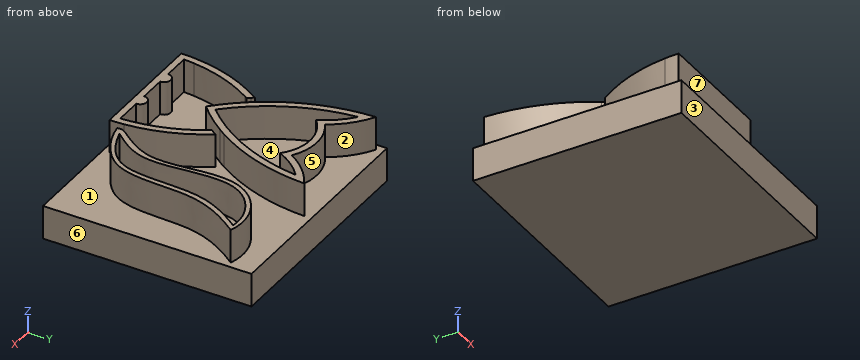
from build123d import *

# Parameters (mm, degrees)
F0_W     = 40
F0_H     = 40
F1_DEPTH = 5
F3_DEPTH = 5
F5_DEPTH = 5
F7_DEPTH = 5


with BuildPart() as f1:
    # F0 (on Top) → F1 (new body)
    with BuildSketch(Plane.XY):
        with Locations((0, -1.4423078379)):
            Rectangle(F0_W, F0_H)
    extrude(amount=F1_DEPTH)

    # F2 (on face) → F3 (join)
    with BuildSketch(Plane.XY.offset(5)):
        with BuildLine():
            ThreePointArc((-14.1666666667, 12.7937878067), (-16.2497421132, 15.4842249108), (-18.9811853554, 17.5132327819))
            ThreePointArc((-18.9811853554, 17.5132327819), (-17.6558893012, 9.8311930383), (-14.3321956463, 2.7797247698))
            ThreePointArc((-14.3321956463, 2.7797247698), (-14.0384410091, 2.335690009), (-13.7365842266, 1.8971228665))
            ThreePointArc((-13.7365842266, 1.8971228665), (-11.9756652837, -0.3650490595), (-10, -2.4423078379))
            ThreePointArc((-10, -2.4423078379), (-8.0243347163, -0.3650490595), (-6.2634157734, 1.8971228665))
            ThreePointArc((-6.2634157734, 1.8971228665), (-5.9615589909, 2.335690009), (-5.6678043537, 2.7797247698))
            ThreePointArc((-5.6678043537, 2.7797247698), (-2.3441106988, 9.8311930383), (-1.0188146446, 17.5132327819))
            ThreePointArc((-1.0188146446, 17.5132327819), (-3.7502578868, 15.4842249108), (-5.8333333333, 12.7937878067))
            ThreePointArc((-5.8333333333, 12.7937878067), (-10, 14.0576921621), (-14.1666666667, 12.7937878067))
        make_face()
        with BuildLine():
            ThreePointArc((-17.8386090668, 15.5557186069), (-15.9104422617, 13.6025441919), (-14.5, 11.2481079219))
            ThreePointArc((-14.5, 11.2481079219), (-10, 13.0576921621), (-5.5, 11.2481079219))
            ThreePointArc((-5.5, 11.2481079219), (-4.0895577383, 13.6025441919), (-2.1613909332, 15.5557186069))
            ThreePointArc((-2.1613909332, 15.5557186069), (-4.6538444684, 6.6592721087), (-9.9058957618, -0.9417174409))
            ThreePointArc((-9.9058957618, -0.9417174409), (-9.952889806, -0.9900282388), (-10, -1.0382257802))
            ThreePointArc((-10, -1.0382257802), (-10.047110194, -0.9900282388), (-10.0941042382, -0.9417174409))
            ThreePointArc((-10.0941042382, -0.9417174409), (-15.3461555316, 6.6592721087), (-17.8386090668, 15.5557186069))
        make_face(mode=Mode.SUBTRACT)
        with BuildLine():
            ThreePointArc((-14.6746917604, 1.49429313), (-14.813143454, 1.6962594848), (-14.9499420607, 1.8993491722))
            ThreePointArc((-14.9499420607, 1.8993491722), (-17.6333766655, -3.4591843441), (-18.9055769047, -9.3154808935))
            ThreePointArc((-18.9055769047, -9.3154808935), (-18.9763826057, -10.3778468743), (-19, -11.4423078379))
            Line((-19, -11.4423078379), (-18, -11.4423078379))
            Line((-18, -11.4423078379), (-2, -11.4423078379))
            Line((-2, -11.4423078379), (-1, -11.4423078379))
            ThreePointArc((-1, -11.4423078379), (-1.0236173943, -10.3778468743), (-1.0944230953, -9.3154808935))
            ThreePointArc((-1.0944230953, -9.3154808935), (-2.3666233345, -3.4591843441), (-5.0500579393, 1.8993491722))
            ThreePointArc((-5.0500579393, 1.8993491722), (-5.186856546, 1.6962594848), (-5.3253082396, 1.49429313))
            ThreePointArc((-5.3253082396, 1.49429313), (-5.4938586481, 1.2530963551), (-5.664766687, 1.0135643809))
            ThreePointArc((-5.664766687, 1.0135643809), (-5.5400096968, 0.8177401798), (-5.4172359122, 0.6206665334))
            ThreePointArc((-5.4172359122, 0.6206665334), (-3.2558828795, -3.9460840787), (-2.1437824802, -8.8745616111))
            ThreePointArc((-2.1437824802, -8.8745616111), (-2.0693638619, -9.6573915088), (-2.0217494138, -10.4423078379))
            Line((-2.0217494138, -10.4423078379), (-6, -10.4423078379))
            ThreePointArc((-6, -10.4423078379), (-7, -9.4423078379), (-8, -10.4423078379))
            Line((-8, -10.4423078379), (-12, -10.4423078379))
            ThreePointArc((-12, -10.4423078379), (-13, -9.4423078379), (-14, -10.4423078379))
            Line((-14, -10.4423078379), (-17.9782505862, -10.4423078379))
            ThreePointArc((-17.9782505862, -10.4423078379), (-17.9306361381, -9.6573915088), (-17.8562175198, -8.8745616111))
            ThreePointArc((-17.8562175198, -8.8745616111), (-16.7441171205, -3.9460840787), (-14.5827640878, 0.6206665334))
            ThreePointArc((-14.5827640878, 0.6206665334), (-14.4599903032, 0.8177401798), (-14.335233313, 1.0135643809))
            ThreePointArc((-14.335233313, 1.0135643809), (-14.5061413519, 1.2530963551), (-14.6746917604, 1.49429313))
        make_face()
    extrude(amount=F3_DEPTH)

    # F4 (on face) → F5 (join)
    with BuildSketch(Plane.XY.offset(5)):
        with BuildLine():
            add(Edge.make_bspline(
                [(0.122830745, -9.643862473), (0.0800776075, -9.2564371629), (-0.2836475293, -8.6528840078), (6.0697106921, -2.7539463587), (0.1924889118, 11.010617472), (8.8871559228, 16.3315651176), (13.0897243609, 14.9395701919)],
                knots=[0, 0, 0, 0, 0.0892731935, 0.3389697324, 0.6872592966, 1, 1, 1, 1], degree=3))
            add(Edge.make_bspline(
                [(0.122830745, -9.643862473), (2.0720909999, -9.4130289317), (10.0156728008, -6.4074475552), (7.6737975893, 6.9160370202), (11.3169839092, 12.5534842645), (13.0897243609, 14.9395701919)],
                knots=[0, 0, 0, 0, 0.3064110943, 0.6750197333, 1, 1, 1, 1], degree=3))
        make_face()
        with BuildLine():
            add(Edge.make_bspline(
                [(1.0569917504, -8.7510244921), (3.4597109512, -8.0260629747), (9.0131155024, -5.6121363011), (7.0344823054, 7.3072493213), (10.3734166024, 12.3634970165), (12.0017683264, 14.648278338)],
                knots=[0, 0, 0, 0, 0.2977508402, 0.6737539057, 1, 1, 1, 1], degree=3))
            add(Edge.make_bspline(
                [(12.0017683264, 14.648278338), (9.1677881113, 15.1552440171), (1.2156290574, 11.3124895915), (6.3737009511, -3.1480270391), (2.0842432148, -7.4958972715), (1.0569917504, -8.7510244921)],
                knots=[0, 0, 0, 0, 0.3213012994, 0.7197281403, 1, 1, 1, 1], degree=3))
        make_face(mode=Mode.SUBTRACT)
    extrude(amount=F5_DEPTH)

    # F6 (on face) → F7 (cut, through all)
    with BuildSketch(Plane.XY.offset(5)):
        Polygon((-20, -21.4423078379), (20, -21.4423078379), (20, 18.5576921621), (14, 18.5576921621), (14, -12.4423078379), (-20, -12.4423078379), align=None)
    extrude(amount=-F7_DEPTH, mode=Mode.SUBTRACT)


solid = f1.part
The model under review builds one solid part; all positions refer to its coordinate system, in mm. Face numbers are marked on the shaded views. A direction names the side the tool comes from. Round coordinates to 2 decimals unless told otherwise and drop trailing zeros. Order: outer loops, then holes, each group sorted by start corner. A loop starts at its lowest first (then second) coordinate and runs counter-clockwise, first axis right, second up. Notation, with made-up numbers: (-21, 82.25) -> (-12, 82.25) arc R13 ccw to (-12, 92.25) -> close; hole circle Ø11 at (-13.5, 46). An arc over 180 degrees is marked (long way). Use CSV: the item, a comma, the result in double quotes. Start each with the question number.
(1) Wall thickness on probe 1 along X at (y, z) = (-2, 7.25); probe 2 along Z at (x, y) = (-15, -1.5); probe 3 along X at (y, z) = (6.5, 7.5): over which ranges is each line inside the solid? List them lowest first. Write a range as from..to.
(2) Mouldability with a two-part tool opening along Y and no side actions: class the marked faces 1, 2, 3 and 4 as pulls with the +Y half, pulls with the -Y half, needs draft (parallel to the pull), parting line crosses it, or undercut.
(3) Tool access review of the marked faces 5, 6 and 7: name each direction out of +Z, -Z, +X, -X, +Y, -Y from which nothing blocks a thin tool from reaching the whole face with its end or side.
(4) Consider section B-B on x = -13. Write out the cut boundary in (y, z), and give its area (3 significant figures).
(5) Insertion check: pin 1 (3 mm diameter, centred on x = -4.5, z = 7.5, fed in from +Y); pin 2 (2 mm diameter, centred on y = 10, z = 8.5, fed in from -X); pin 3 (2 mm diameter, centred on x = -16.5, z = 8.5, fed in from +Y). Each pin has a flat end and moves straight along its axis. Give the tip position at first contact, or say it passes through.
(6) Consider section A-A on z = 6.25. State how many separate pieces and enclosed holes the cut face has, and give its area (3 significant figures).
Responses:
1,probe 1,"-17.06..-15.97, -10.45..-9.55, -4.03..-2.94, 3.68..4.4, 7.75..8.49"
1,probe 2,"0..5"
1,probe 3,"-16.37..-15.27, -4.73..-3.63, 3.13..3.82, 8.25..9.06"
2,face 1,"undercut"
2,face 2,"pulls with the +Y half"
2,face 3,"pulls with the -Y half"
2,face 4,"undercut"
3,face 5,"+Z, +Y"
3,face 6,"+Z, -Z, +X, +Y, -Y"
3,face 7,"+Z, +X, -X, -Y"
4,outline,"(-12.44, 0) -> (18.56, 0) -> (18.56, 5) -> (13.43, 5) -> (13.43, 10) -> (12.32, 10) -> (12.32, 5) -> (2.59, 5) -> (2.59, 10) -> (0.89, 10) -> (0.89, 5) -> (-9.44, 5) -> (-9.44, 10) -> (-11.44, 10) -> (-11.44, 5) -> (-12.44, 5) -> close"
4,area,"179 mm²"
5,pin 1,"y = 16.16"
5,pin 2,"x = -18"
5,pin 3,"y = 16.56"
6,separate pieces,"3"
6,enclosed holes,"2"
6,area,"153 mm²"
